Source: CAD feature listing. Evaluate the final solid. Frame: model axes, mm. A direction names the side the tool comes from. Coordinates: 2 decimals unless noted, no trailing zeros. Loops run counter-clockwise (first coordinate to the right, second up) from the corner with the lowest first, then second, coordinate; pieces in that order, holes last. Notation, with made-up numbers: M 14.5,3 L 36.5,3 A30 ccw 36.5,40 Z; hole C 27.5,81.5 d8. An arc over 180 degrees is marked long. One line per question, with ' | ' between items. Start each with the question number.
1. Pin query (flat end, axial travel): P1, Ø6, axis at x = 8, z = -15, coming from the +Y side (3 decimals); P2, Ø2, axis at y = 8, z = -15.5, coming from the +X side; P3, Ø5, axis at x = -16.5, y = 3.5, coming from the -Z side; P4, Ø3, axis at x = -15, z = -1.5, coming from the +Y side. Return the tip coordinate at first contact, or that it passes through.
2. Access query for faces 1 (the flat face through (-18, 0, -3)), 2 (the flat face through (14.7, 7.938, -16.4)). Directions: +Z, -Z, +X, -X, +Y, -Y. A direction counts if a zero-diameter tool reaches every point of the face in a straight line with its end or side. Return the directions, or none.
3. Section query C-C, the plane y = 3. Output: boundary loops of the cut face in (x, z) (3 decimals).
4. Ray query, probe 1 along X at (y, z) = (5.75, 0) (3 decimals); probe 2 along X at (y, z) = (8, -0.5). Return the intervals inside material, ascending.
5. Mould query, pull axis X, two halves, no side actions, for faces 3 (the cylindrical face through (-6.56, 4.81, -20.82)), 4 (the flat face through (14.7, 1.588, -16.4)), 5 (the cylindrical face through (5.31, 4.7, -16.86)). Classes: pulls with the +X half, pulls with the -X half, needs draft (parallel to the pull), parting line crosses it, or undercut.
Autodesk Inventor part; units mm, degrees
ref_plane "YZ Plane" through (0, 0, 0) normal (1, 0, 0) x (0, 1, 0)
ref_plane "XZ Plane" through (0, 0, 0) normal (0, 1, 0) x (-1, 0, 0)
ref_plane "XY Plane" through (0, 0, 0) normal (0, 0, 1) x (1, 0, 0)
sketch "Sketch1" plane through (0, 0, 0) normal (1, 0, 0) x (0, 1, 0)
  line L0 (0, 0) -> (9.525, 0)
  line L1 (9.525, 0) -> (9.525, -17.675)
  line L2 (9.525, -17.675) -> (0, -17.675)
  line L3 (0, -17.675) -> (0, 0)
  line L4 (0, 0) -> (9.525, 0)
  line L5 (9.525, 0) -> (9.525, -22.225)
  line L6 (9.525, -22.225) -> (0, -22.225)
  line L7 (0, -22.225) -> (0, 0)
  line L8 (1.5875, -21.8281) -> (7.9375, -21.8281)
  line L9 (7.9375, -21.8281) -> (7.9375, -22.6219)
  line L10 (7.9375, -22.6219) -> (1.5875, -22.6219) construction
  line L11 (1.5875, -22.6219) -> (1.5875, -21.8281)
  line L12 (1.5875, -21.8281) -> (7.9375, -22.6219) construction
  line L13 (7.9375, -21.8281) -> (1.5875, -22.6219) construction
  point P0 (4.7625, -22.225)
  point P1 (7.9375, -22.225)
  point P2 (0, -17.675)
  point P3 (1.5875, -22.225)
  dimension "d0" = 17.675
  dimension "d1" = 9.525
  dimension "d2" = 22.225
  dimension "d3" = 6.35
  dimension "d4" = 0.7937
revolve "Revolution1" add sketch "Sketch1" angle 360 about axis through (0, 0, 0) along (0, 1, 0) contours L2 L5 L6 L9 L8 L11 L7
chamfer "Chamfer1" distance 0.7937 angle 45 2 edges at (0, 9.525, 22.225) (0, 0, 22.225)
properties part number "Band - Hub" material "Nylon 6/6"
Taken from the geometry:
1) P1: y = 9.525 | P2: x = 16.84 | P3: z = -16.75 | P4: through
2) face 1: +Z, -Z, +X, -X, -Y | face 2: none
3) outline: C 0,0 d43.656; hole C 0,0 d35.35
4) probe 1: -21.828 to -17.675, 17.675 to 21.828 | probe 2: -22.22 to -17.67, 17.67 to 22.22
5) face 3: parting line crosses it | face 4: needs draft | face 5: undercut
